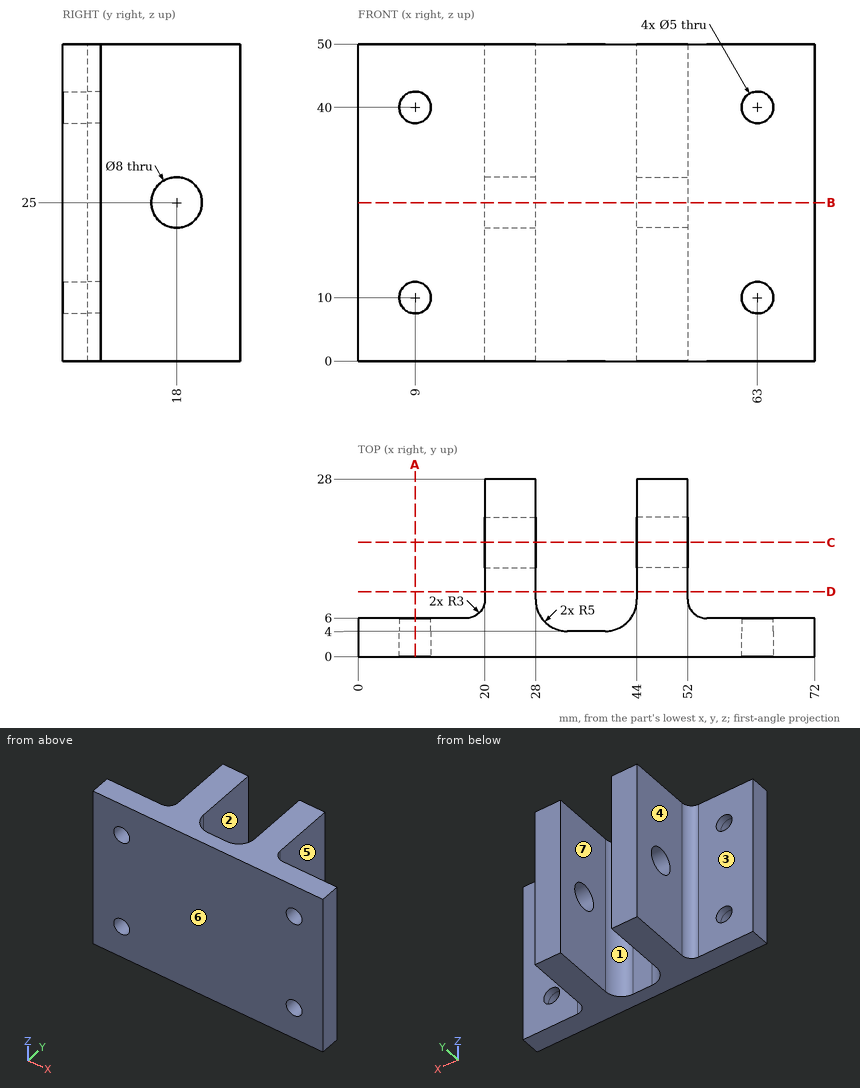
The figure shows three views and two pictorial views of one solid part (mm, origin at its lowest corner). Answer the questions. A direction names the side the tool comes from. Give positions to 0.01 mm unless a question says otherwise; leave off trailing zeros. Order: outer loops, then holes, each group sorted by start corner. A loop starts at its lowest first (then second) coordinate and runs counter-clockwise, first axis right, second up. Notation, with made-up numbers: (-28.5, 36.25) -> (-17.5, 36.25) arc R17 ccw to (-17.5, 61.25) -> close; hole circle Ø11 at (74, -15.5). An arc over 180 degrees is marked (long way). Write each question's results on one line, items separated by ' | '.
Q1. The part is cut by section A-A, the plane x = 9. Give the vertices of the cut face in (y, z).
Checked values:
outline: (0, 0) -> (6, 0) -> (6, 7.5) -> (0, 7.5) -> close; (0, 12.5) -> (6, 12.5) -> (6, 37.5) -> (0, 37.5) -> close; (0, 42.5) -> (6, 42.5) -> (6, 50) -> (0, 50) -> close
Q2. The part is cut by section C-C, the plane y = 18. Give the vertices of the cut face in (x, z), and give its area (3 significant figures).
Checked values:
outline: (20, 0) -> (28, 0) -> (28, 21) -> (20, 21) -> close; (20, 29) -> (28, 29) -> (28, 50) -> (20, 50) -> close; (44, 0) -> (52, 0) -> (52, 21) -> (44, 21) -> close; (44, 29) -> (52, 29) -> (52, 50) -> (44, 50) -> close | area: 672 mm^2
Q3. Each of these flat-tipped pins is pushed along its axis until it touches: P1, Ø4, axis at x = 63, z = 10, coming from the -Y side; P2, Ø1.5, axis at y = 24, z = 33, coming from the +X side; P3, Ø5.5, axis at y = 23, z = 24, coming from the -X side; P4, Ø4, axis at y = 9, z = 12.5, coming from the -X side. Where does it stop, or does it pass through?
Checked values:
P1: passes through | P2: stops at x = 52 | P3: stops at x = 20 | P4: stops at x = 19.24
Q4. Which of the six approach directions +Z, -Z, +X, -X, +Y, -Y give full straight-line access (tool end or side, diameter ignored) to the marked faces 5, 6 and 7?
Checked values:
face 5: +Z, -Z, +X, +Y | face 6: +Z, -Z, +X, -X, -Y | face 7: +Z, -Z, +Y
Q5. Determine the mould class of the marked faces 1, 2, 3 and 4 for opening direction X: pulls with the +X half, pulls with the -X half, needs draft (parallel to the pull), parting line crosses it, or undercut.
Checked values:
face 1: undercut | face 2: undercut | face 3: needs draft | face 4: pulls with the -X half
Q6. The part is cut by section D-D, the plane y = 10.25. Give the vertices of the cut face in (x, z).
Checked values:
outline: (20, 0) -> (28, 0) -> (28, 50) -> (20, 50) -> close; (44, 0) -> (52, 0) -> (52, 50) -> (44, 50) -> close
Q7. The part is cut by section B-B, the plane z = 25. Give the vertices of the cut face in (x, y).
Checked values:
outline: (0, 0) -> (72, 0) -> (72, 6) -> (55, 6) arc R3 cw to (52, 9) -> (52, 14) -> (44, 14) -> (44, 9) arc R5 cw to (39, 4) -> (33, 4) arc R5 cw to (28, 9) -> (28, 14) -> (20, 14) -> (20, 9) arc R3 cw to (17, 6) -> (0, 6) -> close; (20, 22) -> (28, 22) -> (28, 28) -> (20, 28) -> close; (44, 22) -> (52, 22) -> (52, 28) -> (44, 28) -> close
Q8. Straight lines are drawn through the part: probe 1 along Z at (x, y) = (9, 3.2); probe 2 along X at (y, z) = (2.9, 40); probe 3 along X at (y, z) = (19.5, 47.5). For each, find the intervals that lie inside material, in ascending order. Write a range as from..to.
Checked values:
probe 1: z = 0..7.5, 12.5..37.5, 42.5..50 | probe 2: x = 0..6.5, 11.5..60.5, 65.5..72 | probe 3: x = 20..28, 44..52
